Can you work these out from the model? Positions are in its coordinate system, mm. A direction names the side the tool comes from. Give positions to 0.01 mm unless a question says otherwise; leave off trailing zeros. Order: outer loops, then holes, each group sorted by start corner. A loop starts at its lowest first (then second) coordinate and runs counter-clockwise, first axis right, second up. Notation, with made-up numbers: (9.5, -33.75) - (46.5, -33.75) arc R19 cw to (46.5, -19.75) - close; hole circle Ø8 at (84.5, 70.5). An arc over 180 degrees is marked (long way). Use one line per item in the form item = value. Start each with the question number.
1) Please list where this line runs through material, in increasing order: probe 1 along Y at (x, z) = (38.5, 391).
2) Suppose I cut it at A-A, the plane z = 346. Write out the boundary of the cut face in (x, y), and give its area (3 significant figures).
3) We'd pull the mould along Z, two halves only. Please class faces 4 (the flat face through (-1, 13, 0)), 5 (the cylindrical face through (-0.783, 24.775, 387.855)), 6 (the flat face through (25, 0, 213)): released by +Z, released by -Z, zero draft, split by the parting line, or undercut.
4) Suppose I cut it at B-B, the plane z = 398.5. Write out the boundary of the cut face in (x, y).
5) For pin 1 (10 mm diameter, centred on y = 24.77, z = 29.54, fed in from -X); pin 2 (24.5 mm diameter, centred on y = 36, z = 124.5, fed in from +X); pin 3 (24.5 mm diameter, centred on x = 14, z = 237, fed in from +Y), each with a flat end and sliding along its axis, tell me the tip position at first contact or that it passes through.
6) Which directions (+Z, -Z, +X, -X, +Y, -Y) give clear straight access to the entire face, cutting with the end or side of a thin tool? Please do faces 1 (the flat face through (0, 24, 213)), 2 (the flat face through (-1, 13, 431.8)), 3 (the cylindrical face through (-0.78, 25.39, 236.73)).
7) Suppose I cut it at C-C, the plane x = 45. Write out the boundary of the cut face in (y, z), and give its area (3 significant figures).
```python
from build123d import *

# Parameters (mm, degrees)
BOSS_EXTRUDE2_DEPTH = 431.8
CUT_EXTRUDE3_DEPTH  = 127
SKETCH7_R           = 3.175
CUT_EXTRUDE4_DEPTH  = 127


with BuildPart() as part:
    # Sketch3 → Boss-Extrude2 (new body)
    with BuildSketch(Plane.XY):
        Polygon((0, 0), (0, 49.2125), (-1.5875, 49.2125), (-1.5875, -1.5875), (49.2125, -1.5875), (49.2125, 0), align=None)
    extrude(amount=BOSS_EXTRUDE2_DEPTH)

    # Sketch6 → Cut-Extrude3 (cut)
    with BuildSketch(Plane(origin=(0, 0, 0), x_dir=(0, 0, -1), z_dir=(1, 0, 0))):
        with BuildLine():
            Line((-373.888, 39.0525), (-250.698, 39.0525))
            ThreePointArc((-250.698, 39.0525), (-236.728, 25.0825), (-250.698, 11.1125))
            Line((-250.698, 11.1125), (-373.888, 11.1125))
            ThreePointArc((-373.888, 11.1125), (-387.858, 25.0825), (-373.888, 39.0525))
        make_face()
    extrude(amount=-CUT_EXTRUDE3_DEPTH, mode=Mode.SUBTRACT)

    # Sketch7 → Cut-Extrude4 (cut)
    with BuildSketch(Plane(origin=(0, 0, 0), x_dir=(0, 0, -1), z_dir=(1, 0, 0))):
        with Locations((-29.538792285, 24.773594829)):
            Circle(SKETCH7_R)
    extrude(amount=-CUT_EXTRUDE4_DEPTH, mode=Mode.SUBTRACT)


solid = part.part
```
Result sheet:
q1.probe_1 = -1.59 to 0
q2.outline = (-1.59, -1.59) - (49.21, -1.59) - (49.21, 0) - (0, 0) - (0, 11.11) - (-1.59, 11.11) - close; (-1.59, 39.05) - (0, 39.05) - (0, 49.21) - (-1.59, 49.21) - close
q2.area = 114 mm²
q3.face_4 = released by -Z
q3.face_5 = undercut
q3.face_6 = zero draft
q4.outline = (-1.59, -1.59) - (49.21, -1.59) - (49.21, 0) - (0, 0) - (0, 49.21) - (-1.59, 49.21) - close
q5.pin_1 = -1.59
q5.pin_2 = 0
q5.pin_3 = 0
q6.face_1 = +Z, -Z, +X, +Y
q6.face_2 = +Z, +X, -X, +Y, -Y
q6.face_3 = +X, -X
q7.outline = (-1.59, 0) - (0, 0) - (0, 431.8) - (-1.59, 431.8) - close
q7.area = 685 mm²
